from build123d import *

# Parameters (mm, degrees)
F0_R     = 6.35
F0_R_2   = 3.81
F1_DEPTH = 6.35
F2_W     = 1.27
F2_H     = 1.27
F3_DEPTH = 6.35
F4_R     = 0.635


with BuildPart() as f1:
    # F0 (on Top) → F1 (new body)
    with BuildSketch(Plane.XY):
        Circle(F0_R)
        Circle(F0_R_2, mode=Mode.SUBTRACT)
    extrude(amount=F1_DEPTH)

    # F2 (on face) → F3 (join)
    with BuildSketch(Plane.XY.offset(6.35)):
        Polygon((25.4, -5.08), (25.4, 5.08), (5.08, 5.08), (5.08, 3.81), (3.81, 3.81), (3.81, -3.81), (5.08, -3.81), (5.08, -5.08), align=None)
        Polygon((3.81, 5.08), (5.08, 5.08), (5.08, 25.4), (-5.08, 25.4), (-5.08, 5.08), (-3.81, 5.08), (-3.81, 3.81), (3.81, 3.81), align=None)
        with Locations((4.445, 4.445)):
            Rectangle(F2_W, F2_H)
        Polygon((5.08, -25.4), (5.08, -5.08), (3.81, -5.08), (3.81, -3.81), (-3.81, -3.81), (-3.81, -5.08), (-5.08, -5.08), (-5.08, -25.4), align=None)
        with Locations((4.445, -4.445)):
            Rectangle(F2_W, F2_H)
        with Locations((-4.445, 4.445)):
            Rectangle(F2_W, F2_H)
        Polygon((-3.81, -3.81), (-3.81, 3.81), (-5.08, 3.81), (-5.08, 5.08), (-25.4, 5.08), (-25.4, -5.08), (-5.08, -5.08), (-5.08, -3.81), align=None)
        with Locations((-4.445, -4.445)):
            Rectangle(F2_W, F2_H)
    extrude(amount=-F3_DEPTH)

    # F4
    f4_edges = [f1.edges().sort_by_distance(p)[0] for p in [
        (-3.81, 0, 6.35),
        (-3.81, 0, 0),
        (-15.24, -5.08, 0),
        (-5.08, -15.24, 0),
        (0, -25.4, 0),
        (5.08, -15.24, 0),
        (15.24, -5.08, 0),
        (25.4, 0, 0),
        (15.24, 5.08, 0),
        (5.08, 15.24, 0),
        (0, 25.4, 0),
        (-5.08, 15.24, 0),
        (-15.24, 5.08, 0),
        (-25.4, 0, 0),
        (-15.24, -5.08, 6.35),
        (-5.08, -15.24, 6.35),
        (0, -25.4, 6.35),
        (5.08, -15.24, 6.35),
        (15.24, -5.08, 6.35),
        (25.4, 0, 6.35),
        (15.24, 5.08, 6.35),
        (5.08, 15.24, 6.35),
        (0, 25.4, 6.35),
        (-5.08, 15.24, 6.35),
        (-15.24, 5.08, 6.35),
        (-25.4, 0, 6.35),
    ]]
    fillet(f4_edges, radius=F4_R)


solid = f1.part
Verification items for the finished model (mm, model axes). A direction names the side the tool comes from. Coordinates: 2 decimals unless noted, no trailing zeros. Order: outer loops, then holes, each group sorted by start corner. A loop starts at its lowest first (then second) coordinate and runs counter-clockwise, first axis right, second up. Notation, with made-up numbers: (-19, 44.25) -> (20, 44.25) arc R32 cw to (20, 78.25) -> close; hole circle Ø8 at (-17, -22.5). An arc over 180 degrees is marked (long way). Put each result on its own line as item: value. Start each with the question number.
1. Cross-section at C-C, the plane z = 3.25. Record the boundary of the cut face in (x, y).
2. Go/stop test with flat-tipped pins: pin 1 Ø1 at (y, z) = (6.5, 1.5) entering from +X; pin 2 Ø2.5 at (y, z) = (-16, 2.5) entering from -X; pin 3 Ø1.5 at (x, z) = (-10, 2) entering from +Y. Record where each tip stops, or that it passes through.
3. Cross-section at A-A, the plane x = 0. Record the boundary of the cut face in (y, z) (3 decimals).
4. Mould release check, pull along Y, two halves, no side actions. Record for faces 1 (the flat face through (25.4, 0, 3)), 2 (the cylindrical face through (-0.83, -3.72, 3.14)), 3 (the flat face through (-15, -5.08, 3)): released by +Y, released by -Y, zero draft, split by the parting line, or undercut.
5. Material ranges on L1, parallel to Y at x = 0, z = 2.2; L2, parallel to Y at x = -14, z = 4.5, recorded low to high. Write a range as [from, to].
6. Access from +Z, -Z, +X, -X, +Y, -Y to the whole of each face (thin tool, end or side, straight path). Record for faces 4 (the flat face through (-15, 5.08, 3)), 5 (the flat face through (-5.08, -15, 3)), 6 (the flat face through (5.08, 15, 3)).
7. Cross-section at D-D, the plane y = -7. Record the boundary of the cut face in (x, z) (3 decimals), then the cut area to 3 significant figures.
Computed:
1. outline: (-25.4, -5.08) -> (-5.08, -5.08) -> (-5.08, -25.4) -> (5.08, -25.4) -> (5.08, -5.08) -> (25.4, -5.08) -> (25.4, 5.08) -> (5.08, 5.08) -> (5.08, 25.4) -> (-5.08, 25.4) -> (-5.08, 5.08) -> (-25.4, 5.08) -> close; hole circle Ø7.62 at (0, 0)
2. pin 1: x = 5.08
2. pin 2: x = -5.08
2. pin 3: y = 5.08
3. outline: (-25.4, 0.635) arc R0.635 ccw to (-24.765, 0) -> (-4.445, 0) arc R0.635 ccw to (-3.81, 0.635) -> (-3.81, 5.715) arc R0.635 ccw to (-4.445, 6.35) -> (-24.765, 6.35) arc R0.635 ccw to (-25.4, 5.715) -> close; (3.81, 0.635) arc R0.635 ccw to (4.445, 0) -> (24.765, 0) arc R0.635 ccw to (25.4, 0.635) -> (25.4, 5.715) arc R0.635 ccw to (24.765, 6.35) -> (4.445, 6.35) arc R0.635 ccw to (3.81, 5.715) -> close
4. face 1: zero draft
4. face 2: undercut
4. face 3: released by -Y
5. L1: [-25.4, -3.81], [3.81, 25.4]
5. L2: [-5.08, 5.08]
6. face 4: +Z, -Z, -X, +Y
6. face 5: +Z, -Z, -X, -Y
6. face 6: +Z, -Z, +X, +Y
7. outline: (-5.08, 0.635) arc R0.635 ccw to (-4.445, 0) -> (4.445, 0) arc R0.635 ccw to (5.08, 0.635) -> (5.08, 5.715) arc R0.635 ccw to (4.445, 6.35) -> (-4.445, 6.35) arc R0.635 ccw to (-5.08, 5.715) -> close
7. area: 64.2 mm2
